Autodesk Inventor part; units mm, degrees
ref_plane "YZ Plane" through (0, 0, 0) normal (1, 0, 0) x (0, 1, 0)
ref_plane "XZ Plane" through (0, 0, 0) normal (0, 1, 0) x (-1, 0, 0)
ref_plane "XY Plane" through (0, 0, 0) normal (0, 0, 1) x (1, 0, 0)
sketch "スケッチ1" plane through (0, 0, 0) normal (0, 1, 0) x (-1, 0, 0)
  circle A0 centre (0, 0) radius 3
  circle A1 centre (0, 0) radius 6
  dimension "d0" = 6
  dimension "d1" = 12
extrude "押し出し1" add sketch "スケッチ1" along normal blind 5
fillet "フィレット1" radius 0.5 1 edges at (6, 5, 0)
fillet "フィレット2" radius 0.5 1 edges at (6, 0, 0)
properties part number "セットカラー 内径6 外径12 幅5" material "アルミニウム 6061"
Part model, mm, in its own coordinate system. Round coordinates to 2 decimals unless told otherwise and drop trailing zeros. Order: outer loops, then holes, each group sorted by start corner. A loop starts at its lowest first (then second) coordinate and runs counter-clockwise, first axis right, second up. Notation, with made-up numbers: (22.5, -1.5) -> (73.5, -1.5) arc R30 cw to (73.5, 33.5) -> close; hole circle Ø5 at (1, -8). An arc over 180 degrees is marked (long way). Put each result on its own line as item: value.
Q1. Pin check, flat tips, straight feed: pin 1 Ø5.5 at (x, z) = (0, 0) entering from +Y; pin 2 Ø1.5 at (x, y) = (1.5, 4) entering from +Z; pin 3 Ø1.5 at (x, y) = (-4.5, 4) entering from +Z; pin 4 Ø3 at (y, z) = (3, -2.5) entering from +X. Stop position of each tip, or through.
From the geometry:
pin 1: passes through
pin 2: stops at z = 5.95
pin 3: stops at z = 4.68
pin 4: stops at x = 5.92
Q2. Band-saw the part on B-B (x = 0). Give the cut face in (y, z), and give its area (3 significant figures).
From the geometry:
outline: (0, -5.5) arc R0.5 ccw to (0.5, -6) -> (4.5, -6) arc R0.5 ccw to (5, -5.5) -> (5, -3) -> (0, -3) -> close; (0, 3) -> (5, 3) -> (5, 5.5) arc R0.5 ccw to (4.5, 6) -> (0.5, 6) arc R0.5 ccw to (0, 5.5) -> close
area: 29.8 mm2
Q3. Pull direction X, two halves, no side cores. Call faces 1 (the face through (3, 2, 0)), 2 (the face through (6, 2, 0)), 3 (the face through (-2.4, 5, -2.4)): pulls with the +X half, pulls with the -X half, needs draft (parallel to the pull), parting line crosses it, or undercut.
From the geometry:
face 1: undercut
face 2: parting line crosses it
face 3: needs draft
Q4. Band-saw the part on A-A (z = 0). Give the cut face in (x, y).
From the geometry:
outline: (-6, 0.5) arc R0.5 ccw to (-5.5, 0) -> (-3, 0) -> (-3, 5) -> (-5.5, 5) arc R0.5 ccw to (-6, 4.5) -> close; (3, 0) -> (5.5, 0) arc R0.5 ccw to (6, 0.5) -> (6, 4.5) arc R0.5 ccw to (5.5, 5) -> (3, 5) -> close
Q5. Wall check: line 1 (Z direction, x = 0, y = 2.65); line 2 (Z direction, x = -1.75, y = 1.3); line 3 (X direction, y = 4.5, z = -2.75). Give the ranges that are in metal, low to high. Write a range as [from, to].
From the geometry:
line 1: z = [-6, -3], [3, 6]
line 2: z = [-5.74, -2.44], [2.44, 5.74]
line 3: x = [-5.33, -1.2], [1.2, 5.33]
Q6. Band-saw the part on C-C (y = 2.7). Give the cut face in (x, z), and give its area (3 significant figures).
From the geometry:
outline: circle Ø12 at (0, 0); hole circle Ø6 at (0, 0)
area: 84.8 mm2
